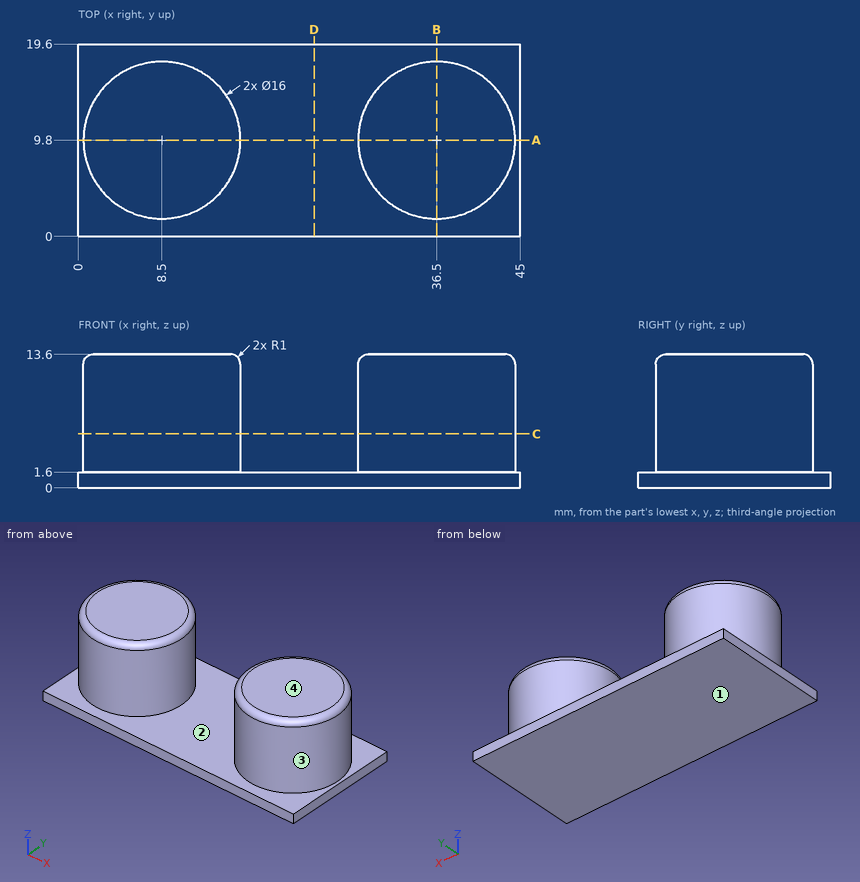
Check sheet for the drawn part. Datum: minimum x, y, z corner. Units: mm. A direction names the side the tool comes from. Coordinates: 2 decimals unless noted, no trailing zeros. Loops run counter-clockwise (first coordinate to the right, second up) from the corner with the lowest first, then second, coordinate; pieces in that order, holes last. Notation, with made-up numbers: (58.25, 50.25) - (86.25, 50.25) arc R28 cw to (86.25, 69.25) - close; hole circle Ø8 at (-15, 40). An arc over 180 degrees is marked (long way). Put each result on its own line as item: value.
Item 1: Section check D-D (x = 24). Enter the section's corners in (y, z).
Conclusion:
outline: (0, 0) - (19.6, 0) - (19.6, 1.6) - (0, 1.6) - close
Item 2: Section check B-B (x = 36.5). Enter the section's corners in (y, z), then the cut area to 3 significant figures.
Conclusion:
outline: (0, 0) - (19.6, 0) - (19.6, 1.6) - (17.8, 1.6) - (17.8, 12.6) arc R1 ccw to (16.8, 13.6) - (2.8, 13.6) arc R1 ccw to (1.8, 12.6) - (1.8, 1.6) - (0, 1.6) - close
area: 223 mm2
Item 3: Section check C-C (z = 5.5). Enter the section's corners in (x, y), then the cut area to 3 significant figures.
Conclusion:
outline: circle Ø16 at (8.5, 9.8); circle Ø16 at (36.5, 9.8)
area: 402 mm2
Item 4: Scan lines: line 1 along Z through (x, y) = (27, 12.75); line 2 along X through (y, z) = (16, 3); line 3 along X through (y, z) = (11.75, 2). Record each from-to range of solid material in increasing order.
Conclusion:
line 1: z = 0 to 1.6
line 2: x = 3.44 to 13.56, 31.44 to 41.56
line 3: x = 0.74 to 16.26, 28.74 to 44.26
Item 5: Set-up check for the marked faces 1 and 2: record each of +Z, -Z, +X, -X, +Y, -Y from which the full face is reachable in a straight line by a thin tool's end or side.
Conclusion:
face 1: -Z, +X, -X, +Y, -Y
face 2: +Z
Item 6: Draft check along X on the marked faces 3 and 4. Enter one of: pulls with the +X half, pulls with the -X half, needs draft (parallel to the pull), parting line crosses it, or undercut.
Conclusion:
face 3: undercut
face 4: needs draft
Item 7: Gauge pin test, flat ends, axial feed: pin 1 Ø1 at (x, z) = (5.5, 7.5) entering from +Y; pin 2 Ø6 at (x, y) = (25, 8.5) entering from +Z; pin 3 Ø2 at (y, z) = (2.5, 9) entering from +X. Record the tip position at first contact, or that the pin passes through.
Conclusion:
pin 1: stops at y = 17.4
pin 2: stops at z = 1.6
pin 3: stops at x = 41.43
Item 8: Section check A-A (y = 9.8). Enter the section's corners in (x, z).
Conclusion:
outline: (0, 0) - (45, 0) - (45, 1.6) - (44.5, 1.6) - (44.5, 12.6) arc R1 ccw to (43.5, 13.6) - (29.5, 13.6) arc R1 ccw to (28.5, 12.6) - (28.5, 1.6) - (16.5, 1.6) - (16.5, 12.6) arc R1 ccw to (15.5, 13.6) - (1.5, 13.6) arc R1 ccw to (0.5, 12.6) - (0.5, 1.6) - (0, 1.6) - close
